Part model, mm, in its own coordinate system. A direction names the side the tool comes from. Give positions to 0.01 mm unless a question says otherwise; leave off trailing zeros. Write each loop counter-clockwise with the first axis right and the second up, starting at its lowest first coordinate (ties: lowest second). Pieces come first, ordered by that corner, then holes. Notation, with made-up numbers: M 61,-12.75 L 113,-12.75 A23 ccw 113,9.25 Z; hole C -15.5,23.25 d7. An arc over 180 degrees is marked long. Use a Markdown table: item, result. Add a question column.
from build123d import *

# Parameters (mm, degrees)
SKETCH1_W               = 120
SKETCH1_H               = 110
SKETCH1_W_2             = 2
SKETCH1_H_2             = 50
BOSS_EXTRUDE1_DEPTH     = 5
SKETCH2_R               = 1.55
CUT_EXTRUDE1_DEPTH      = 82.547532152
CROQUIS1_W              = 57.6
CROQUIS1_H              = 41
SALIENTE_EXTRUIR1_DEPTH = 7.5
CROQUIS3_W              = 34.20218154
CROQUIS3_H              = 8.093357641
CORTAR_EXTRUIR1_DEPTH   = 132.328633588
CROQUIS4_R              = 1.3
CORTAR_EXTRUIR2_DEPTH   = 98.283361887
REDONDEO1_R             = 30
CHAFL_N1_SIZE           = 2
CHAFL_N2_SIZE           = 2
CHAFL_N3_SIZE           = 1
REDONDEO2_R             = 1
CROQUIS5_W              = 30.259884699
CROQUIS5_H              = 22.835005582
CORTAR_EXTRUIR3_DEPTH   = 82.79549155


with BuildPart() as part:
    # Sketch1 → Boss-Extrude1 (new body)
    with BuildSketch(Plane(origin=(0, 0, 0), x_dir=(1, 0, 0), z_dir=(0, 1, 0))):
        Rectangle(SKETCH1_W, SKETCH1_H)
        Rectangle(SKETCH1_W_2, SKETCH1_H_2, mode=Mode.SUBTRACT)
    extrude(amount=BOSS_EXTRUDE1_DEPTH)

    # Sketch2 → Cut-Extrude1 (cut, through all)
    with BuildSketch(Plane(origin=(0, 5, 0), x_dir=(1, 0, 0), z_dir=(0, 1, 0))):
        with Locations(Location((9, 28, 0), (0, 0, 270))):
            Circle(SKETCH2_R)
        with Locations(Location((9, 10, 0), (0, 0, 270))):
            Circle(SKETCH2_R)
        with Locations(Location((27, 10, 0), (0, 0, 270))):
            Circle(SKETCH2_R)
        with Locations(Location((27, 28, 0), (0, 0, 270))):
            Circle(SKETCH2_R)
        with Locations(Location((-24, 46, 0), (0, 0, 270))):
            Circle(SKETCH2_R)
        with Locations(Location((26, 46, 0), (0, 0, 270))):
            Circle(SKETCH2_R)
        with Locations(Location((27, -28, 0), (0, 0, 90))):
            Circle(SKETCH2_R)
        with Locations(Location((27, -10, 0), (0, 0, 90))):
            Circle(SKETCH2_R)
        with Locations(Location((9, -10, 0), (0, 0, 90))):
            Circle(SKETCH2_R)
        with Locations(Location((9, -28, 0), (0, 0, 90))):
            Circle(SKETCH2_R)
        with Locations(Location((26, -46, 0), (0, 0, 90))):
            Circle(SKETCH2_R)
        with Locations(Location((-24, -46, 0), (0, 0, 90))):
            Circle(SKETCH2_R)
        with BuildLine():
            Line((46, 22.4), (62.391060934, 22.4))
            Line((62.391060934, 22.4), (62.391060934, 25.6))
            Line((62.391060934, 25.6), (45.999999974, 25.6))
            ThreePointArc((45.999999974, 25.6), (44.4, 23.999999987), (46, 22.4))
        make_face()
        with BuildLine():
            Line((62.391060934, -25.6), (45.999999974, -25.6))
            ThreePointArc((45.999999974, -25.6), (44.4, -23.999999987), (46, -22.4))
            Line((46, -22.4), (62.391060934, -22.4))
            Line((62.391060934, -22.4), (62.391060934, -25.6))
        make_face()
    extrude(amount=-CUT_EXTRUDE1_DEPTH, mode=Mode.SUBTRACT)

    # Croquis1 → Saliente-Extruir1 (add)
    with BuildSketch(Plane(origin=(0, 5, 0), x_dir=(1, 0, 0), z_dir=(0, 1, 0))):
        with Locations((-29.8, 0.05)):
            Rectangle(CROQUIS1_W, CROQUIS1_H)
    extrude(amount=SALIENTE_EXTRUIR1_DEPTH)

    # Croquis3 → Cortar-Extruir1 (cut, through all)
    with BuildSketch(Plane.ZY.offset(58.6)):
        with Locations((-0.065699517, 8.453321179)):
            Rectangle(CROQUIS3_W, CROQUIS3_H)
    extrude(amount=-CORTAR_EXTRUIR1_DEPTH, mode=Mode.SUBTRACT)

    # Croquis4 → Cortar-Extruir2 (cut, through all)
    with BuildSketch(Plane(origin=(0, 0, -20.55), x_dir=(-1, 0, 0), z_dir=(0, 0, -1))):
        with Locations((31.1, 7.709263706)):
            Circle(CROQUIS4_R)
        with Locations((9.100000064, 7.707582737)):
            Circle(CROQUIS4_R)
    extrude(amount=-CORTAR_EXTRUIR2_DEPTH, mode=Mode.SUBTRACT)

    # Redondeo1
    # the kernel refuses this fillet: 30 mm, written as the material it takes off along each edge
    with BuildSketch(Plane(origin=(60, -74.9849985, -55), x_dir=(-1, 0, 0), z_dir=(0, 1, 0))) as redondeo1_piece_1:
        with BuildLine():
            CenterArc((29.9939994, 30), REDONDEO1_R, 181.145991998, 88.854008002)
            Line((0, 29.4), (-0.599879988, 29.388))
            ThreePointArc((-0.599879988, 29.388), (-0.6, 14.7), (-0.6, 0))
            Line((-0.6, 0), (0, -0.6))
            Line((0, -0.6), (29.9939994, -0.6))
            Line((29.9939994, -0.6), (29.9939994, 0))
        make_face()
    extrude(amount=154.969996999, mode=Mode.SUBTRACT)
    with BuildSketch(Plane(origin=(-60, -75, -55), x_dir=(1, 0, 0), z_dir=(0, 1, 0)), Plane(origin=(-60, -75, 55), x_dir=(0, 0, -1), z_dir=(0, 1, 0))) as redondeo1_piece_2:
        with BuildLine():
            CenterArc((REDONDEO1_R, -REDONDEO1_R), REDONDEO1_R, 90, 90)
            Line((0, -REDONDEO1_R), (-REDONDEO1_R * 0.02, -REDONDEO1_R))
            Line((-REDONDEO1_R * 0.02, -REDONDEO1_R), (-REDONDEO1_R * 0.02, REDONDEO1_R * 0.02))
            Line((-REDONDEO1_R * 0.02, REDONDEO1_R * 0.02), (REDONDEO1_R, REDONDEO1_R * 0.02))
            Line((REDONDEO1_R, REDONDEO1_R * 0.02), (REDONDEO1_R, 0))
        make_face()
    extrude(amount=155, mode=Mode.SUBTRACT)
    with BuildSketch(Plane(origin=(60, -74.9849985, 55), x_dir=(-1, 0, 0), z_dir=(0, 1, 0))) as redondeo1_piece_3:
        with BuildLine():
            CenterArc((29.9939994, -30), REDONDEO1_R, 90, 88.854008002)
            Line((0, -29.4), (-0.599879988, -29.388))
            ThreePointArc((-0.599879988, -29.388), (-0.6, -14.7), (-0.6, 0))
            Line((-0.6, 0), (0, 0.6))
            Line((0, 0.6), (29.9939994, 0.6))
            Line((29.9939994, 0.6), (29.9939994, 0))
        make_face()
    extrude(amount=154.969996999, mode=Mode.SUBTRACT)

    # Chaflán1
    # the kernel refuses this chamfer: 2 mm, written as the material it adds along each edge
    with BuildSketch(Plane(origin=(-1, 5, 20.45), x_dir=(0, -0.02749587661058651, 0.9996219169112968), z_dir=(-1, 0, 0))) as chafl_n1_piece_1_section:
        Polygon((CHAFL_N1_SIZE * 0.999621916911, CHAFL_N1_SIZE * 0.0274958766106), (-CHAFL_N1_SIZE * 0.0274958766106, CHAFL_N1_SIZE * 0.999621916911), (0, 0), align=None)
    chafl_n1_piece_1 = extrude(amount=57.6, mode=Mode.PRIVATE)
    chafl_n1_piece_1 = chafl_n1_piece_1 - Plane(origin=(-31.1, 7.709263706, 21.1121364), x_dir=(-1, 0, 0), z_dir=(0, 0, -1)) * Cylinder(1.3, 124, mode=Mode.PRIVATE)
    chafl_n1_piece_1 = chafl_n1_piece_1 - Plane(origin=(-9.100000064, 7.707582737, 21.1121364), x_dir=(-1, 0, 0), z_dir=(0, 0, -1)) * Cylinder(1.3, 124, mode=Mode.PRIVATE)
    add(chafl_n1_piece_1)
    with BuildSketch(Plane(origin=(-58.6, 5, -20.55), x_dir=(0, -0.02749587661058651, -0.9996219169112968), z_dir=(1, 0, 0))) as chafl_n1_piece_2_section:
        Polygon((CHAFL_N1_SIZE * 0.999621916911, CHAFL_N1_SIZE * 0.0274958766106), (-CHAFL_N1_SIZE * 0.0274958766106, CHAFL_N1_SIZE * 0.999621916911), (0, 0), align=None)
    chafl_n1_piece_2 = extrude(amount=57.6, mode=Mode.PRIVATE)
    chafl_n1_piece_2 = chafl_n1_piece_2 - Plane(origin=(-31.1, 7.709263706, -21.2121364), x_dir=(-1, 0, 0), z_dir=(0, 0, -1)) * Cylinder(1.3, 124, mode=Mode.PRIVATE)
    chafl_n1_piece_2 = chafl_n1_piece_2 - Plane(origin=(-9.100000064, 7.707582737, -21.2121364), x_dir=(-1, 0, 0), z_dir=(0, 0, -1)) * Cylinder(1.3, 124, mode=Mode.PRIVATE)
    add(chafl_n1_piece_2)
    # the kernel refuses this chamfer: 2 mm, written as the material it takes off along each edge
    with BuildSketch(Plane(origin=(-58.6, 12.5, -12.023424311), x_dir=(-0.027495876610585623, -0.9996219169112968, 0), z_dir=(0, 0, -1)), Plane(origin=(-1, 12.5, -25.693365976), x_dir=(0.02749587661058638, -0.9996219169112968, 0), z_dir=(0, 0, 1))) as chafl_n1_2_piece_1:
        Polygon((CHAFL_N1_SIZE * 0.999621916911, -CHAFL_N1_SIZE * 0.0274958766106), (-CHAFL_N1_SIZE * 0.0274958766106, -CHAFL_N1_SIZE * 0.999621916911), (0, 0), align=None)
    extrude(amount=13.669941665, mode=Mode.SUBTRACT)
    with BuildSketch(Plane(origin=(-1, 12.5, 11.892025277), x_dir=(0.02749587661058638, -0.9996219169112968, 0), z_dir=(0, 0, 1)), Plane(origin=(-58.6, 12.5, 25.593365976), x_dir=(-0.027495876610585623, -0.9996219169112968, 0), z_dir=(0, 0, -1))) as chafl_n1_2_piece_2:
        Polygon((CHAFL_N1_SIZE * 0.999621916911, -CHAFL_N1_SIZE * 0.0274958766106), (-CHAFL_N1_SIZE * 0.0274958766106, -CHAFL_N1_SIZE * 0.999621916911), (0, 0), align=None)
    extrude(amount=13.701340699, mode=Mode.SUBTRACT)

    # Chaflán2
    chafl_n2_edges = [part.edges().sort_by_distance(p)[0] for p in [
        (27, 0, 29.55),
        (27, 0, -29.55),
        (27, 0, -11.55),
        (9, 0, -11.55),
        (27, 0, 11.55),
        (9, 0, 11.55),
        (9, 0, 29.55),
        (9, 0, -29.55),
    ]]
    chamfer(chafl_n2_edges, length=CHAFL_N2_SIZE)

    # Chaflán3
    chafl_n3_edges = [part.edges().sort_by_distance(p)[0] for p in [
        (-1, 0, 0),
    ]]
    chamfer(chafl_n3_edges, length=CHAFL_N3_SIZE)
    chafl_n3_2_edges = [part.edges().sort_by_distance(p)[0] for p in [
        (0, 0, 25),
    ]]
    chamfer(chafl_n3_2_edges, length=CHAFL_N3_SIZE)
    chafl_n3_3_edges = [part.edges().sort_by_distance(p)[0] for p in [
        (0, 0, -25),
    ]]
    chamfer(chafl_n3_3_edges, length=CHAFL_N3_SIZE)
    chafl_n3_4_edges = [part.edges().sort_by_distance(p)[0] for p in [
        (1, 0, 0),
    ]]
    chamfer(chafl_n3_4_edges, length=CHAFL_N3_SIZE)
    chafl_n3_5_edges = [part.edges().sort_by_distance(p)[0] for p in [
        (1, 5, 21.017695626),
    ]]
    chamfer(chafl_n3_5_edges, length=CHAFL_N3_SIZE)

    # Redondeo2
    redondeo2_edges = [part.edges().sort_by_distance(p)[0] for p in [
        (60, 2.5, -22.4),
        (60, 2.5, -25.6),
        (60, 2.5, 25.6),
        (60, 2.5, 22.4),
    ]]
    fillet(redondeo2_edges, radius=REDONDEO2_R)

    # Croquis5 → Cortar-Extruir3 (cut, through all)
    with BuildSketch(Plane(origin=(0, 4.406642359, 0), x_dir=(1, 0, 0), z_dir=(0, 1, 0))):
        with Locations((-29.699516464, 0)):
            Rectangle(CROQUIS5_W, CROQUIS5_H)
    extrude(amount=-CORTAR_EXTRUIR3_DEPTH, mode=Mode.SUBTRACT)


solid = part.part
1. Cut at A-A (z = -10). Give the number of separate pieces and of enclosed holes in the cut face, then the cut area to 3 significant figures.
2. Cut at D-D (z = 46). Write the cut outline in (x, y).
3. Tool access for faces 5 (the flat face through (-30, 4.407, -12)), 6 (the flat face through (-30, 2, 11.418)), 7 (the cylindrical face through (50.856, 2.465, -46.571)), 8 (the flat face through (53, 3, -25.6)): list every direction of +Z, -Z, +X, -X, +Y, -Y with a clear straight run to the whole face (end or side of a thin tool).
4. Cut at C-C (x = -16). Write the cut outline in (y, z), then the cut area to 3 significant figures.
5. Mould opens along Z. For faces 1 (the cylindrical face through (8.06, 3.22, -11.23)), 2 (the flat face through (0, 2, 55)), 3 (the flat face through (-30, 2, -11.418)), 4 (the flat face through (-58.6, 8, -19)) say: released by +Z, released by -Z, zero draft, split by the parting line, or undercut.
6. Flat gauge pins, fed straight in: pin 1 (3 mm diameter, centred on x = -45.5, z = 6.5, fed in from -Y); pin 2 (1 mm diameter, centred on x = 30, z = -20.5, fed in from +Y); pin 3 (3.5 mm diameter, centred on x = -9.1, y = 7.71, fed in from +Z); pin 4 (5 mm diameter, centred on x = 9, z = 28, fed in from -Y). Where does each tip first touch, or does it go through?
7. Drill centre lines: probe 1 along X at (y, z) = (2.45, -46); probe 2 along Y at (x, z) = (-9, 20); probe 3 along Z at (x, y) = (-17, 10.75). Where is each one in solid material? Low to high. Write a range as [from, to].
A:
| question | item | result |
|---|---|---|
| 1 | separate pieces | 5 |
| 1 | enclosed holes | 0 |
| 1 | area | 351 mm² |
| 2 | outline | M -51.42,0 L -25.55,0 L -25.55,5 L -51.42,5 Z; M -22.45,0 L 24.45,0 L 24.45,5 L -22.45,5 Z; M 27.55,0 L 51.43,0 L 51.43,5 L 27.55,5 Z |
| 3 | face 5 | +X, +Y |
| 3 | face 6 | +Y, -Y |
| 3 | face 7 | -Z, +X, +Y, -Y |
| 3 | face 8 | +X, +Y, -Y |
| 4 | outline | M 0,-55 L 5,-55 L 5,-22.55 L 7,-20.55 L 12.5,-20.55 L 12.5,-17.17 L 4.41,-17.17 L 4.41,-11.42 L 0,-11.42 Z; M 0,11.42 L 4.41,11.42 L 4.41,17.04 L 12.5,17.04 L 12.5,20.45 L 7,20.45 L 5,22.45 L 5,55 L 0,55 Z |
| 4 | area | 484 mm² |
| 5 | face 1 | undercut |
| 5 | face 2 | released by +Z |
| 5 | face 3 | undercut |
| 5 | face 4 | zero draft |
| 6 | pin 1 | stops at y = 0 |
| 6 | pin 2 | stops at y = 5 |
| 6 | pin 3 | stops at z = 21.49 |
| 6 | pin 4 | stops at y = 1.05 |
| 7 | probe 1 | x = [-51.42, -25.55], [-22.45, 24.45], [27.55, 51.43] |
| 7 | probe 2 | y = [0, 6.41], [9, 12.5] |
| 7 | probe 3 | z = [-20.55, -17.17], [17.04, 20.45] |
